For this review, use the dimensioned drawing (mm, ordinates from the lowest corner) and the shaded views. A direction names the side the tool comes from. Coordinates: 2 decimals unless noted, no trailing zeros. Order: outer loops, then holes, each group sorted by start corner. A loop starts at its lowest first (then second) coordinate and runs counter-clockwise, first axis right, second up. Notation, with made-up numbers: M 18,-28.75 L 49,-28.75 A21 cw 49,-20.75 Z; hole C 17,11.5 d8. An arc over 180 degrees is marked long. Write each question's results on one line, items separated by ' | '.
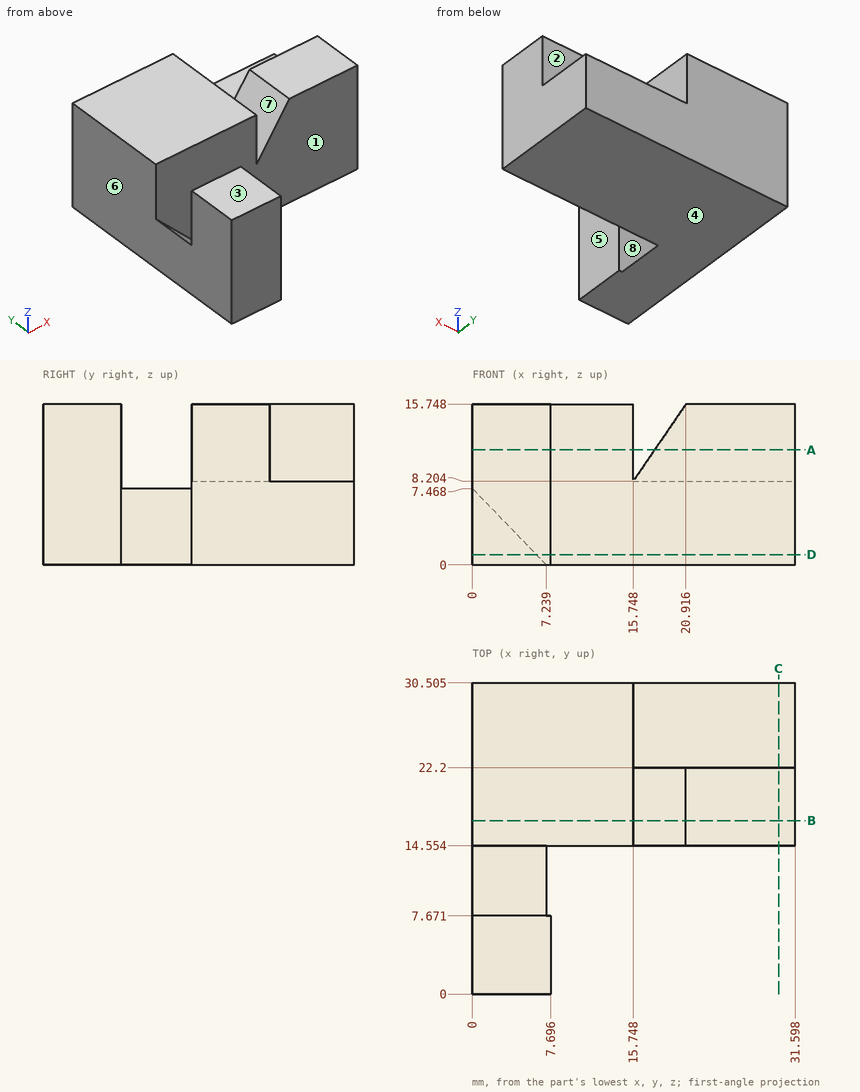
1) Take a section at B-B on y = 17. State the section outline as (x, z) points (1 decimal).
Solutions:
outline: M 0,0 L 31.6,0 L 31.6,15.7 L 20.9,15.7 L 15.7,8.2 L 15.7,15.7 L 0,15.7 Z
2) Take a section at A-A on z = 11.25. State the section outline as (x, y) points (1 decimal).
Solutions:
outline: M 0,0 L 7.7,0 L 7.7,7.7 L 0,7.7 Z; M 0,14.6 L 15.7,14.6 L 15.7,30.5 L 0,30.5 Z; M 17.8,14.6 L 31.6,14.6 L 31.6,22.2 L 17.8,22.2 Z
3) For the marked faces 1, 2, 3, 4 and 5, list the 3-axis set-ups (+Z, -Z, +X, -X, +Y, -Y) from which the entire face can be reached by the end or side of a thin tool; tool diameter is ignored.
Solutions:
face 1: +Z, +X | face 2: +Z, +X, +Y | face 3: +Z, +X, -X, +Y, -Y | face 4: -Z, +X, -X, +Y, -Y | face 5: +Z, -Z, +X, -Y
4) To check wall thickness, follow line 1 along Y through (x, z) = (7.5, 9.5) (1 decimal); line 2 along Y through (x, z) = (18, 9) (1 decimal); line 3 along Y through (x, z) = (9, 12) (1 decimal). State the ranges of each line that lie inside material, in increasing order.
Solutions:
line 1: 0 to 7.7, 14.6 to 30.5 | line 2: 14.6 to 22.2 | line 3: 14.6 to 30.5
5) The part is to be moulded in two halves that separate along X. For the marked faces 6, 7 and 8, say which applies: pulls with the +X half, pulls with the -X half, needs draft (parallel to the pull), parting line crosses it, or undercut.
Solutions:
face 6: pulls with the -X half | face 7: undercut | face 8: needs draft
6) For pin 1 (8 mm diameter, centred on x = 18.5, z = 6.5, fed in from -Y); pin 2 (8.5 mm diameter, centred on x = 24, z = 14, fed in from +Y); pin 3 (6.5 mm diameter, centred on x = 25, y = 27.5, fed in from +Z), all flat-tipped, find the tip position at first contact; note any pin that passes through.
Solutions:
pin 1: y = 14.55 | pin 2: y = 22.2 | pin 3: z = 8.2
7) Take a section at C-C on x = 30. State the section outline as (y, z) points (1 decimal).
Solutions:
outline: M 14.6,0 L 30.5,0 L 30.5,8.2 L 22.2,8.2 L 22.2,15.7 L 14.6,15.7 Z
8) Take a section at D-D on z = 1. State the section outline as (x, y) points (1 decimal).
Solutions:
outline: M 0,0 L 7.7,0 L 7.7,7.7 L 6.3,7.7 L 6.3,14.6 L 31.6,14.6 L 31.6,30.5 L 0,30.5 Z
